from build123d import *

# Parameters (mm, degrees)
SKETCH1_W               = 95
SKETCH1_H               = 72
BOSS_EXTRUDE1_DEPTH     = 35
SKETCH5_W               = 90
SKETCH5_H               = 68
CUT_EXTRUDE1_DEPTH      = 33
SKETCH10_R              = 1
BOSS_EXTRUDE5_DEPTH     = 72
CUT_EXTRUDE2_DEPTH      = 10
CUT_EXTRUDE2_DEPTH_BACK = 3
SKETCH19_W              = 5
SKETCH19_H              = 26
SKETCH20_W              = 90
SKETCH20_H              = 72
CUT_EXTRUDE3_DEPTH      = 3
SKETCH21_R              = 1.5
CUT_EXTRUDE4_DEPTH      = 72.226750593


with BuildPart() as part:
    # Sketch1 → Boss-Extrude1 (new body)
    with BuildSketch(Plane(origin=(0, 0, 0), x_dir=(1, 0, 0), z_dir=(0, 1, 0))):
        Rectangle(SKETCH1_W, SKETCH1_H)
    extrude(amount=BOSS_EXTRUDE1_DEPTH)

    # Sketch5 → Cut-Extrude1 (cut)
    with BuildSketch(Plane(origin=(0, 35, 0), x_dir=(1, 0, 0), z_dir=(0, 1, 0))):
        with Locations((2.5, 0)):
            Rectangle(SKETCH5_W, SKETCH5_H)
    extrude(amount=-CUT_EXTRUDE1_DEPTH, mode=Mode.SUBTRACT)

    # Sketch10 → Boss-Extrude5 (add, through all)
    with BuildSketch(Plane.XY.offset(36)):
        with BuildLine():
            Line((-42.5, 35), (-42.5, 38.5))
            ThreePointArc((-42.5, 38.5), (-45, 41), (-47.5, 38.5))
            Line((-47.5, 38.5), (-47.5, 35))
            Line((-47.5, 35), (-42.5, 35))
        make_face()
        with Locations((-45, 38.5)):
            Circle(SKETCH10_R, mode=Mode.SUBTRACT)
    extrude(amount=-BOSS_EXTRUDE5_DEPTH)

    # Sketch19 → Cut-Extrude2 (cut, two sides: drawn at the far end of the back side and taken through both)
    with BuildSketch(Plane(origin=(0, 35, 0), x_dir=(1, 0, 0), z_dir=(0, 1, 0)).offset(-CUT_EXTRUDE2_DEPTH_BACK)):
        with Locations((-45, -15)):
            Rectangle(SKETCH19_W, SKETCH19_H)
    extrude(amount=CUT_EXTRUDE2_DEPTH + CUT_EXTRUDE2_DEPTH_BACK, mode=Mode.SUBTRACT)

    # Sketch20 → Cut-Extrude3 (cut)
    with BuildSketch(Plane(origin=(0, 35, 0), x_dir=(1, 0, 0), z_dir=(0, 1, 0))):
        with Locations((2.5, 0)):
            Rectangle(SKETCH20_W, SKETCH20_H)
    extrude(amount=-CUT_EXTRUDE3_DEPTH, mode=Mode.SUBTRACT)

    # Sketch21 → Cut-Extrude4 (cut, through all)
    with BuildSketch(Plane(origin=(0, 2, 0), x_dir=(1, 0, 0), z_dir=(0, 1, 0))):
        with Locations(Location((0, 0, 0), (0, 0, 270))):
            Circle(SKETCH21_R)
    extrude(amount=-CUT_EXTRUDE4_DEPTH, mode=Mode.SUBTRACT)


solid = part.part
Could you check a few things on this model? Use its own coordinates, in mm. A direction names the side the tool comes from. Coordinates: 2 decimals unless noted, no trailing zeros. Write each loop counter-clockwise with the first axis right and the second up, starting at its lowest first coordinate (ties: lowest second). Pieces come first, ordered by that corner, then holes. Notation, with made-up numbers: (-5.5, 23) - (24.5, 23) arc R10 ccw to (24.5, 29) - close; hole circle Ø9 at (47, 65). An arc over 180 degrees is marked (long way). Write item = value, one per line.
1) Suppose I cut it at D-D on x = 41.5. Please give me the cut outline in (y, z), plus the area to 3 significant figures.
Result set:
outline = (0, -36) - (32, -36) - (32, -34) - (2, -34) - (2, 34) - (32, 34) - (32, 36) - (0, 36) - close
area = 264 mm2
2) Please list where these lines run through material, in increasing order: line 1 (Z direction, x = 11.5, y = 8); line 2 (Y direction, x = -45, z = -21); line 3 (X direction, y = 30, z = 13). Write a range as [from, to].
Result set:
line_1 = [-36, -34], [34, 36]
line_2 = [0, 37.5], [39.5, 41]
line_3 = [-47.5, -42.5]
3) Will these pins go through, and if not, where does the flat tip stop? pin 1 Ø4 at (y, z) = (32.5, -27) entering from +X; pin 2 Ø1.5 at (x, z) = (-44, 19.5) entering from +Y.
Result set:
pin_1 = -42.5
pin_2 = 32
4) Suppose I cut it at C-C on y = 5.5. Please give me the cut outline in (x, z), plus the area to 3 significant figures.
Result set:
outline = (-47.5, -36) - (47.5, -36) - (47.5, -34) - (-42.5, -34) - (-42.5, 34) - (47.5, 34) - (47.5, 36) - (-47.5, 36) - close
area = 720 mm2
5) We'd pull the mould along Z, two halves only. Please class faces 1 (the flat face through (-1, 16, -36)), 2 (the flat face through (2, 17, 34)), 3 (the flat face through (-1, 0, -9)): +Z half, -Z half, draft (parallel to the pull), parting line (faces both ways), or undercut.
Result set:
face_1 = -Z half
face_2 = undercut
face_3 = draft
6) For faces 4 (the flat face through (2, 17, -34)), 5 (the flat face through (-45, 32, 15)), 6 (the flat face through (2, 32, 35)), which set-ups out of +Z, -Z, +X, -X, +Y, -Y let a thin tool reach every point of the face, with its end or its side?
Result set:
face_4 = +X, +Y
face_5 = +X, -X, +Y
face_6 = +Z, -Z, +X, +Y
7) Suppose I cut it at A-A on z = 0. Please give me the cut outline in (x, y), plus the area to 3 significant figures.
Result set:
outline = (-47.5, 0) - (-1.5, 0) - (-1.5, 2) - (-42.5, 2) - (-42.5, 38.5) arc R2.5 ccw to (-47.5, 38.5) - close; (1.5, 0) - (47.5, 0) - (47.5, 2) - (1.5, 2) - close; hole circle Ø2 at (-45, 38.5)
area = 373 mm2
8) Suppose I cut it at B-B on x = 0. Please give me the cut outline in (y, z), plus the area to 3 significant figures.
Result set:
outline = (0, -36) - (32, -36) - (32, -34) - (2, -34) - (2, -1.5) - (0, -1.5) - close; (0, 1.5) - (2, 1.5) - (2, 34) - (32, 34) - (32, 36) - (0, 36) - close
area = 258 mm2
